Work out the finished part from the listing and answer in its coordinate system (mm). A direction names the side the tool comes from. Give positions to 0.01 mm unless a question says otherwise; leave off trailing zeros. Loops run counter-clockwise (first coordinate to the right, second up) from the corner with the lowest first, then second, coordinate; pieces in that order, holes last. Notation, with made-up numbers: (82, 26.5) - (92, 26.5) arc R35 ccw to (92, 63.5) - close; hole circle Ø8 at (89.25, 72). An arc over 180 degrees is marked (long way). Use one line per item in the form item = value. Start each with the question number.
from build123d import *

# Parameters (mm, degrees)
F2_R     = 5.2
F2_R_2   = 4
F3_DEPTH = 3
F4_R     = 5.15
F4_R_2   = 4.05
F5_DEPTH = 2.95


with BuildPart() as f1:
    # F0 (on Front) → F1 (revolve)
    with BuildSketch(Plane.XZ):
        Polygon((3, 4), (3, 0), (6.8, 0), (6.8, 0.8), (6, 0.8), (6, 4), align=None)
    revolve(axis=Axis((0, 0, 2), (0, 0, 1)))

    # F2 (on face) → F3 (cut)
    with BuildSketch(Plane.XY.offset(4)):
        Circle(F2_R)
        Circle(F2_R_2, mode=Mode.SUBTRACT)
    extrude(amount=-F3_DEPTH, mode=Mode.SUBTRACT)

    # F4 (on face) → F5 (join)
    with BuildSketch(Plane.XY.offset(1)):
        Circle(F4_R)
        Circle(F4_R_2, mode=Mode.SUBTRACT)
    extrude(amount=F5_DEPTH)


solid = f1.part
1) A cutting plane is placed at D-D (y = 3.5). Give the vertices of the cut face in (x, z), plus the area to 3 significant figures.
2) A cutting plane is placed at B-B (x = 0). Give the vertices of the cut face in (y, z).
3) Determine the mould class of faces 1 (the flat face through (4, -5, 0.8)), 2 (the flat face through (-3, -3, 3.95)), 3 (the cylindrical face through (-1.47, -6.64, 0.41)) for opening direction X: released by +X, released by -X, zero draft, split by the parting line, or undercut.
4) Find the intervals of material crossed by probe 1 along Z at (x, y) = (-4, -2.5); probe 2 along Z at (x, y) = (3.25, -5.5); probe 3 along Y at (x, z) = (0, 0.55), in increasing order.
5) A tool of negligible diameter and unlimited length cuts with its end or side. For faces 4 (the cylindrical face through (-3, 0, 2)), 5 (the cylindrical face through (-6, 0, 2)), from which of +Z, -Z, +X, -X, +Y, -Y can it reach the whole face along a straight path? Write none if from no direction.
6) A cutting plane is placed at A-A (z = 2.65). Give the vertices of the cut face in (x, y).
Answer sheet:
q1.outline = (-5.83, 0) - (5.83, 0) - (5.83, 0.8) - (4.87, 0.8) - (4.87, 4) - (3.85, 4) - (3.85, 1) - (3.78, 1) - (3.78, 3.95) - (2.04, 3.95) - (2.04, 1) - (1.94, 1) - (1.94, 4) - (-1.94, 4) - (-1.94, 1) - (-2.04, 1) - (-2.04, 3.95) - (-3.78, 3.95) - (-3.78, 1) - (-3.85, 1) - (-3.85, 4) - (-4.87, 4) - (-4.87, 0.8) - (-5.83, 0.8) - close
q1.area = 39.3 mm²
q2.outline = (-6.8, 0) - (-3, 0) - (-3, 4) - (-4, 4) - (-4, 1) - (-4.05, 1) - (-4.05, 3.95) - (-5.15, 3.95) - (-5.15, 1) - (-5.2, 1) - (-5.2, 4) - (-6, 4) - (-6, 0.8) - (-6.8, 0.8) - close; (3, 0) - (6.8, 0) - (6.8, 0.8) - (6, 0.8) - (6, 4) - (5.2, 4) - (5.2, 1) - (5.15, 1) - (5.15, 3.95) - (4.05, 3.95) - (4.05, 1) - (4, 1) - (4, 4) - (3, 4) - close
q3.face_1 = zero draft
q3.face_2 = undercut
q3.face_3 = split by the parting line
q4.probe_1 = 0 to 3.95
q4.probe_2 = 0 to 0.8
q4.probe_3 = -6.8 to -3, 3 to 6.8
q5.face_4 = +Z, -Z
q5.face_5 = +Z
q6.outline = circle Ø12 at (0, 0); circle Ø10.3 at (0, 0); circle Ø8 at (0, 0); hole circle Ø10.4 at (0, 0); hole circle Ø8.1 at (0, 0); hole circle Ø6 at (0, 0)
